Autodesk Inventor part; units mm, degrees
ref_plane "YZ Plane" through (0, 0, 0) normal (1, 0, 0) x (0, 1, 0)
ref_plane "XZ Plane" through (0, 0, 0) normal (0, 1, 0) x (-1, 0, 0)
ref_plane "XY Plane" through (0, 0, 0) normal (0, 0, 1) x (1, 0, 0)
sketch "Sketch1" plane through (0, 0, 0) normal (1, 0, 0) x (0, 1, 0)
  line L0 (228.6, 215.9) -> (-228.6, 215.9)
  line L1 (-228.6, 215.9) -> (-228.6, -215.9)
  line L2 (-228.6, -215.9) -> (228.6, -215.9)
  line L3 (228.6, -215.9) -> (228.6, 215.9)
  point P0 (0, 0)
  dimension "d0" = 431.8
  dimension "d1" = 457.2
  dimension "d2" = 215.9
  dimension "d3" = 228.6
extrude "Extrusion1" add sketch "Sketch1" along normal mid plane 1092.2
sketch "Sketch2" plane through (546.1, 0, 0) normal (1, 0, 0) x (0, 0, -1)
  line L0 (-38.1, 203.2) -> (12.7, 203.2)
  line L1 (12.7, 203.2) -> (12.7, 0)
  line L2 (12.7, 0) -> (-38.1, 0)
  line L3 (-38.1, 0) -> (-38.1, 203.2)
  line L4 (-215.9, 228.6) -> (-215.9, -228.6)
  line L5 (-215.9, 228.6) -> (215.9, 228.6)
  point P0 (0, 0)
  dimension "d6" = 50.8
  dimension "d7" = 203.2
  dimension "d8" = 228.6
  dimension "d9" = 25.4
extrude "Extrusion2" add sketch "Sketch2" along normal blind 228.6
mirror "Mirror1" about plane through (0, 0, 0) normal (1, 0, 0) of "Extrusion2"
sketch "Sketch3" plane through (546.1, 0, 38.1) normal (0, 0, 1) x (1, 0, 0)
  circle A0 centre (114.3, 101.6) radius 38.1
  line L0 (0, 228.6) -> (0, -228.6)
  line L1 (0, 203.2) -> (228.6, 203.2)
  point P0 (-546.1, 0)
  dimension "d12" = 76.2
  dimension "d13" = 114.3
  dimension "d14" = 101.6
extrude "Extrusion3" cut sketch "Sketch3" against normal through all
mirror "Mirror2" about plane through (0, 0, 0) normal (1, 0, 0) of "Extrusion3"
fillet "Fillet1" radius 50.8 8 edges at (774.7, 203.2, 12.7) (774.7, 0, 12.7) (546.1, 228.6, 0) (546.1, -228.6, 0) (-546.1, 228.6, 0) (-546.1, -228.6, 0) (-774.7, 203.2, 12.7) (-774.7, 0, 12.7)
sketch "Sketch4" plane through (-495.3, -228.6, 215.9) normal (0, 0, 1) x (1, 0, 0)
  circle A0 centre (495.3, 228.6) radius 165.1
  dimension "d18" = 330.2
extrude "Extrusion4" cut sketch "Sketch4" against normal blind 101.6
sketch "Sketch5" plane through (-495.3, -228.6, 215.9) normal (0, 0, 1) x (1, 0, 0)
  line L0 (990.6, 457.2) -> (0, 457.2)
  line L1 (0, 0) -> (990.6, 0)
  line L2 (228.6, 457.2) -> (762, 457.2)
  line L3 (762, 457.2) -> (762, 0)
  line L4 (762, 0) -> (228.6, 0)
  line L5 (228.6, 0) -> (228.6, 457.2)
  line L6 (1041.4, 406.4) -> (1041.4, 50.8)
  line L7 (-50.8, 50.8) -> (-50.8, 406.4)
  point P0 (495.3, 228.6)
  dimension "d21" = 279.4
  dimension "d22" = 279.4
extrude "Extrusion5" cut sketch "Sketch5" against normal blind 50.8
properties part number "Speaker"
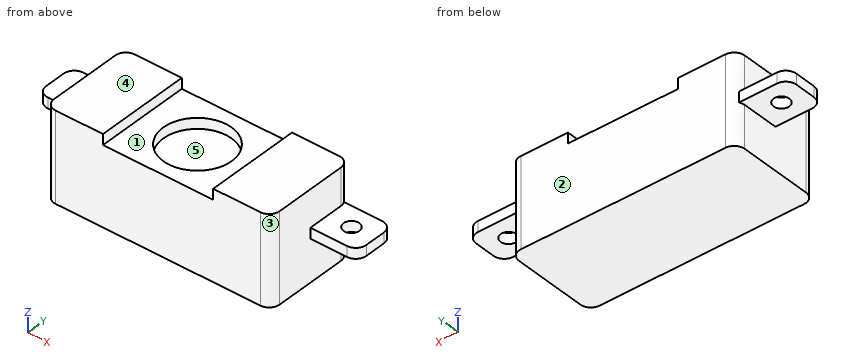
Work out the finished part from the listing and answer in its coordinate system (mm). Face numbers are marked on the shaded views. A direction names the side the tool comes from. Give positions to 0.01 mm unless a question says otherwise; leave off trailing zeros. Loops run counter-clockwise (first coordinate to the right, second up) from the corner with the lowest first, then second, coordinate; pieces in that order, holes last. Notation, with made-up numbers: (-2, -27) -> (57, -27) arc R31 cw to (57, 10) -> close; hole circle Ø10 at (-38.75, -24). An arc over 180 degrees is marked (long way). One line per question, with ' | ' between items. Start each with the question number.
1) Section A-A, the plane z = 15.5 is taken. Determine the outline of the cut face in (x, y).
2) Determine the mould class of the marked faces 1, 2 and 3 for opening direction X: +X half, -X half, draft (parallel to the pull), parting line (faces both ways), or undercut.
3) Straight lines are drawn through the part: L1, parallel to Y at x = 660.4, z = 8; L2, parallel to X at y = -126.5, z = 184.5; L3, parallel to Z at x = -213, y = 13.5. For each, find the intervals that lie inside material, in ascending order.
4) For the marked faces 4 and 5, determine the directions among +Z, -Z, +X, -X, +Y, -Y from which every point of the face is accessible in a straight line to the end or side of a thin tool.
5) Section C-C, the plane z = 132 is taken. Determine the outline of the cut face in (x, y), then the cut area to 3 significant figures.
6) Section D-D, the plane x = 0 is taken. Determine the outline of the cut face in (y, z), then the cut area to 3 significant figures.
7) Each of these flat-tipped pins is pushed along its axis until it touches: pin 1 (8 mm diameter, centred on y = -154.5, z = 159.5, fed in from -X); pin 2 (3 mm diameter, centred on y = 25, z = 153.5, fed in from +X); pin 3 (1 mm diameter, centred on y = -182.5, z = 131, fed in from -X). Where does it stop, or does it pass through?
8) Section B-B, the plane x = 660.4 is taken. Determine the outline of the cut face in (y, z).
Resolved:
1) outline: (-774.7, 50.8) arc R50.8 ccw to (-723.9, 0) -> (-546.1, 0) -> (-546.1, -177.8) arc R50.8 ccw to (-495.3, -228.6) -> (495.3, -228.6) arc R50.8 ccw to (546.1, -177.8) -> (546.1, 0) -> (723.9, 0) arc R50.8 ccw to (774.7, 50.8) -> (774.7, 152.4) arc R50.8 ccw to (723.9, 203.2) -> (539.29, 203.2) arc R50.8 ccw to (495.3, 228.6) -> (-495.3, 228.6) arc R50.8 ccw to (-539.29, 203.2) -> (-723.9, 203.2) arc R50.8 ccw to (-774.7, 152.4) -> close; hole circle Ø76.2 at (-660.4, 101.6); hole circle Ø76.2 at (660.4, 101.6)
2) face 1: undercut | face 2: draft | face 3: +X half
3) L1: 0 to 63.5, 139.7 to 203.2 | L2: -546.1 to -266.7, 266.7 to 546.1 | L3: -215.9 to 165.1
4) face 4: +Z, +X, -X, +Y, -Y | face 5: +Z
5) outline: (-546.1, -177.8) arc R50.8 ccw to (-495.3, -228.6) -> (495.3, -228.6) arc R50.8 ccw to (546.1, -177.8) -> (546.1, 177.8) arc R50.8 ccw to (495.3, 228.6) -> (-495.3, 228.6) arc R50.8 ccw to (-546.1, 177.8) -> close; hole circle Ø330.2 at (0, 0) | area: 412,000 mm2
6) outline: (-228.6, -215.9) -> (228.6, -215.9) -> (228.6, 165.1) -> (165.1, 165.1) -> (165.1, 114.3) -> (-165.1, 114.3) -> (-165.1, 165.1) -> (-228.6, 165.1) -> close | area: 157,000 mm2
7) pin 1: x = -546.1 | pin 2: x = 546.1 | pin 3: x = -545.93
8) outline: (0, -12.7) -> (63.5, -12.7) -> (63.5, 38.1) -> (0, 38.1) -> close; (139.7, -12.7) -> (203.2, -12.7) -> (203.2, 38.1) -> (139.7, 38.1) -> close
